Job drawing, mm, ordinate dimensions from the low corner. One solid piece. A direction names the side the tool comes from. Give positions to 0.01 mm unless a question says otherwise; leave off trailing zeros. Order: outer loops, then holes, each group sorted by start corner. A loop starts at its lowest first (then second) coordinate and runs counter-clockwise, first axis right, second up. Notation, with made-up numbers: (-36.5, 72) -> (7.5, 72) arc R27 cw to (7.5, 99) -> close; hole circle Ø8 at (36, 49.5). An arc over 180 degrees is marked (long way). Write item = value, one per line. Start each with the question number.
(1) Two-plate mould, pull along X, no slides. Class the marked faces 3, 4 and 5: pulls with the +X half, pulls with the -X half, needs draft (parallel to the pull), parting line crosses it, or undercut.
(2) Saw through at C-C, the plane y = 28. List the corners of the cut face in (x, z).
(3) Saw through at A-A, the plane x = 85. List the corners of the cut face in (y, z), then the cut area to 3 significant figures.
(4) Saw through at B-B, the plane y = 42. List the corners of the cut face in (x, z).
(5) Probe line 1 along X through (y, z) = (2, 20); line 2 along X through (y, z) = (58.5, 2.5); line 3 along Y through (x, z) = (165, 20). List the from-to ranges inside material, lowest first. Write a range as from..to.
(6) Flat gauge pins, fed straight in: pin 1 (20 mm diameter, centred on x = 90, z = 15.5, fed in from +Y); pin 2 (4.5 mm diameter, centred on x = 85, z = 20, fed in from -Y). Where does each tip first touch, or does it go through?
(7) Which spindle directions (+Z, -Z, +X, -X, +Y, -Y) get a long thin tool onto all of the face, cutting with end or side? Do the marked faces 1 and 2. Say none if no direction does.
(8) Saw through at D-D, the plane y = 60. List the corners of the cut face in (x, z).
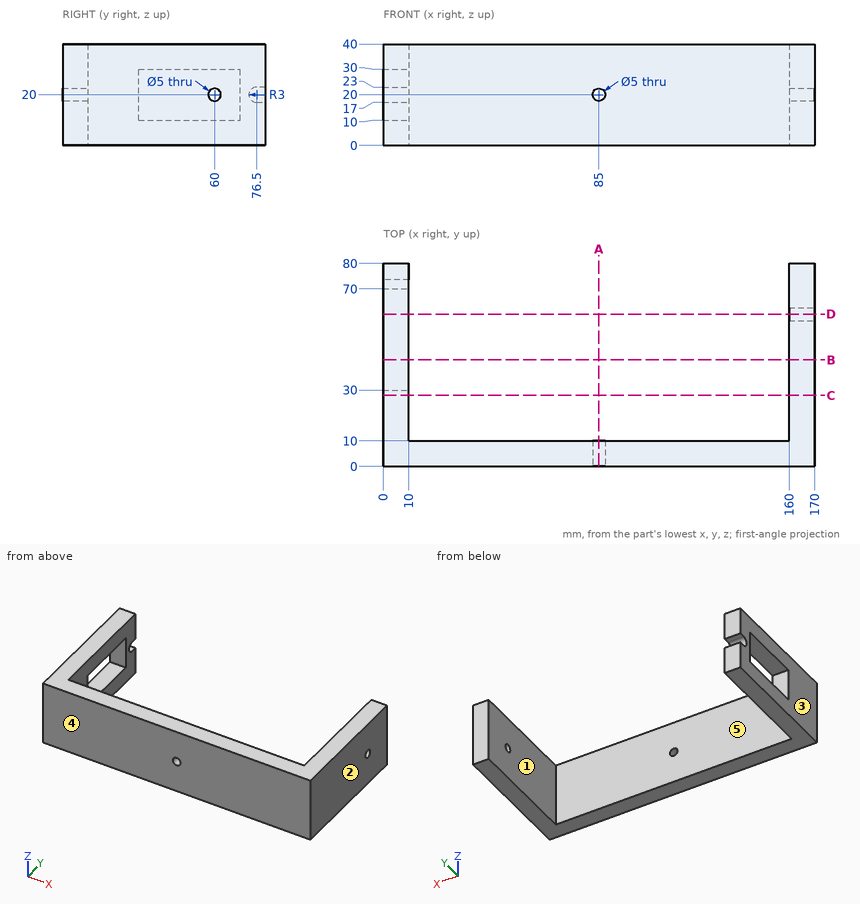
Results list:
q1.face_3 = pulls with the -X half
q1.face_4 = needs draft
q1.face_5 = undercut
q2.outline = (0, 0) -> (10, 0) -> (10, 40) -> (0, 40) -> close; (160, 0) -> (170, 0) -> (170, 40) -> (160, 40) -> close
q3.outline = (0, 0) -> (10, 0) -> (10, 17.5) -> (0, 17.5) -> close; (0, 22.5) -> (10, 22.5) -> (10, 40) -> (0, 40) -> close
q3.area = 350 mm^2
q4.outline = (0, 0) -> (10, 0) -> (10, 10) -> (0, 10) -> close; (0, 30) -> (10, 30) -> (10, 40) -> (0, 40) -> close; (160, 0) -> (170, 0) -> (170, 40) -> (160, 40) -> close
q5.line_1 = 0..82.5, 87.5..170
q5.line_2 = 0..10, 160..170
q5.line_3 = 0..57.5, 62.5..80
q6.pin_1 = 10
q6.pin_2 = through
q7.face_1 = +Z, -Z, +Y
q7.face_2 = +Z, -Z, +X, +Y, -Y
q8.outline = (0, 0) -> (10, 0) -> (10, 10) -> (0, 10) -> close; (0, 30) -> (10, 30) -> (10, 40) -> (0, 40) -> close; (160, 0) -> (170, 0) -> (170, 17.5) -> (160, 17.5) -> close; (160, 22.5) -> (170, 22.5) -> (170, 40) -> (160, 40) -> close
